Model file for the job. Use its own axes, mm. Round coordinates to 2 decimals unless told otherwise and drop trailing zeros. Order: outer loops, then holes, each group sorted by start corner. A loop starts at its lowest first (then second) coordinate and runs counter-clockwise, first axis right, second up. Notation, with made-up numbers: (54, 10) - (66, 10) arc R17 cw to (66, 19) - close; hole circle Ø1 at (13, 42). An arc over 180 degrees is marked (long way). Use one line per item in the form item = value.
from build123d import *

# Parameters (mm, degrees)
MODEL_R            = 1
BOSS_EXTRU_1_DEPTH = 1.6


with BuildPart() as part:
    # Model → Boss.-Extru.1 (new body)
    with BuildSketch(Plane.XY):
        Polygon((98.150595456, 11.331634302), (152.811395456, 25.971686302), (138.282595456, 80.221514302), (78.010935456, 64.541586302), (-24.588554544, 5.301674302), (-151.608757489, 5.292943326), (-172.373873722, 5.291515997), (-172.373873722, -50.687645053), (-172.373873722, -50.858487698), (-9.398592544, -50.858487698), align=None)
        with Locations((-114.030844544, -32.493525698)):
            Circle(MODEL_R, mode=Mode.SUBTRACT)
        with Locations((-10.652844544, -46.438125698)):
            Circle(MODEL_R, mode=Mode.SUBTRACT)
        with Locations((-114.259444544, -13.418125698)):
            Circle(MODEL_R, mode=Mode.SUBTRACT)
        with Locations((-29.702844544, -2.648525698)):
            Circle(MODEL_R, mode=Mode.SUBTRACT)
        with Locations((92.877555456, 28.085474302)):
            Circle(MODEL_R, mode=Mode.SUBTRACT)
        with Locations((80.685555456, 58.489274302)):
            Circle(MODEL_R, mode=Mode.SUBTRACT)
    extrude(amount=BOSS_EXTRU_1_DEPTH)


solid = part.part
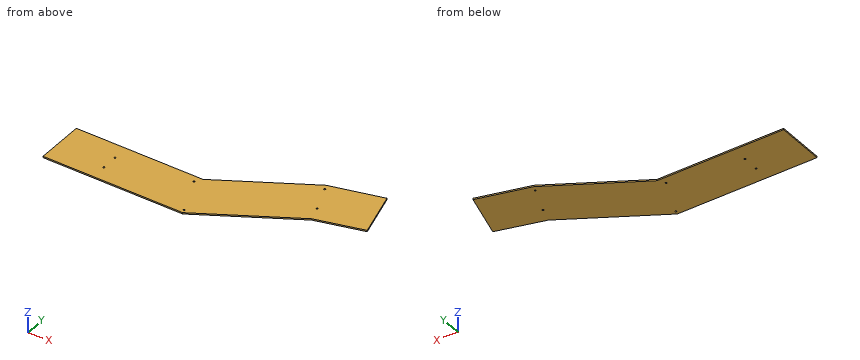
(1) Pin check, flat tips, straight feed: pin 1 (2.5 mm diameter, centred on x = -114.26, y = -13.42, fed in from +Z); pin 2 (1.8 mm diameter, centred on x = 80.69, y = 58.49, fed in from -Z); pin 3 (0.5 mm diameter, centred on x = -166, z = 1, fed in from +Y). Stop position of each tip, or through.
Report:
pin_1 = 1.6
pin_2 = through
pin_3 = 5.29
(2) Slice it at B-B on x = -3.5. Give the cut face in (y, z).
Report:
outline = (-47.45, 0) - (17.48, 0) - (17.48, 1.6) - (-47.45, 1.6) - close
(3) Slice it at C-C on y = 32. Give the cut face in (x, z).
Report:
outline = (21.65, 0) - (151.2, 0) - (151.2, 1.6) - (21.65, 1.6) - close
(4) Probe probe 1 along X at (y, z) = (-13, 1.1); probe 2 along Y at (x, z) = (-72, 0.25); probe 3 along X at (y, z) = (-3, 1.5). List the from-to ranges inside material, lowest first. Write a range as [from, to].
Report:
probe_1 = [-172.37, -115.17], [-113.35, 56.07]
probe_2 = [-50.86, 5.3]
probe_3 = [-172.37, -30.64], [-28.77, 73.37]
(5) Slice it at A-A on z = 1.35. Give the cut face in (x, y).
Report:
outline = (-172.37, -50.86) - (-9.4, -50.86) - (98.15, 11.33) - (152.81, 25.97) - (138.28, 80.22) - (78.01, 64.54) - (-24.59, 5.3) - (-172.37, 5.29) - close; hole circle Ø2 at (-114.26, -13.42); hole circle Ø2 at (-114.03, -32.49); hole circle Ø2 at (-29.7, -2.65); hole circle Ø2 at (-10.65, -46.44); hole circle Ø2 at (80.69, 58.49); hole circle Ø2 at (92.88, 28.09)
